Autodesk Inventor part; units mm, degrees
ref_plane "YZ Plane" through (0, 0, 0) normal (1, 0, 0) x (0, 1, 0)
ref_plane "XZ Plane" through (0, 0, 0) normal (0, 1, 0) x (-1, 0, 0)
ref_plane "XY Plane" through (0, 0, 0) normal (0, 0, 1) x (1, 0, 0)
sketch "Sketch1" plane through (0, 0, 0) normal (0, 0, 1) x (1, 0, 0)
  circle A0 centre (0, 0) radius 5
  arc A1 (-13, 15) -> (-15, 13) centre (-13, 13) ccw
  arc A2 (-15, -13) -> (-13, -15) centre (-13, -13) ccw
  arc A3 (13, -15) -> (15, -13) centre (13, -13) ccw
  arc A4 (15, 13) -> (13, 15) centre (13, 13) ccw
  arc A5 (-13, 14) -> (-14, 13) centre (-13, 13) ccw
  arc A6 (-14, -13) -> (-13, -14) centre (-13, -13) ccw
  arc A7 (13, -14) -> (14, -13) centre (13, -13) ccw
  arc A8 (14, 13) -> (13, 14) centre (13, 13) ccw
  line L0 (14, -14) -> (-14, 14) construction
  line L1 (-14, -14) -> (14, 14) construction
  line L2 (15, -15) -> (-15, 15) construction
  line L3 (-15, -15) -> (15, 15) construction
  line L4 (-13, 15) -> (-8, 15)
  line L5 (-8, 13) -> (-8, 8) construction
  line L6 (-9.4142, 8) -> (-13, 8)
  line L7 (-15, 8) -> (-15, 13)
  line L8 (-13, -15) -> (-8, -15)
  line L9 (-8, -13) -> (-8, -9.4142)
  line L10 (-9.4142, -8) -> (-13, -8)
  line L11 (-15, -8) -> (-15, -13)
  line L12 (13, -15) -> (8, -15)
  line L13 (8, -13) -> (8, -9.4142)
  line L14 (9.4142, -8) -> (13, -8)
  line L15 (15, -8) -> (15, -13)
  line L16 (13, 15) -> (8, 15)
  line L17 (8, 13) -> (8, 9.4142)
  line L18 (9.4142, 8) -> (13, 8)
  line L19 (15, 8) -> (15, 13)
  line L20 (-13, 9) -> (-10, 9)
  line L21 (-9, 10) -> (-9, 13)
  line L22 (-10, 14) -> (-13, 14)
  line L23 (-14, 13) -> (-14, 10)
  line L24 (13, 9) -> (10, 9)
  line L25 (9, 10) -> (9, 13)
  line L26 (10, 14) -> (13, 14)
  line L27 (14, 13) -> (14, 10)
  line L28 (13, -9) -> (10, -9)
  line L29 (9, -10) -> (9, -13)
  line L30 (10, -14) -> (13, -14)
  line L31 (14, -13) -> (14, -10)
  line L32 (-13, -9) -> (-10, -9)
  line L33 (-9, -10) -> (-9, -13)
  line L34 (-10, -14) -> (-13, -14)
  line L35 (-14, -13) -> (-14, -10)
  line L36 (-14, 13) -> (-14, 10)
  line L37 (-14, -10) -> (-14, -13)
  line L38 (-14, -13) -> (-14, -10)
  line L39 (-14, 10) -> (-14, 13)
  line L40 (13, -15) -> (5, -15)
  line L41 (-5, -15) -> (-13, -15)
  line L42 (13, -15) -> (5, -15) construction
  line L43 (0, -15) -> (-13, -15) construction
  line L44 (4, -13) -> (8, -13)
  line L45 (-8, -13) -> (-4, -13)
  line L46 (10, -9) -> (13, -9)
  line L47 (14, -10) -> (14, -13)
  line L48 (13, -14) -> (10, -14)
  line L49 (9, -13) -> (9, -10)
  line L50 (5, -14) -> (5, -15)
  line L51 (13, -14) -> (10, -14)
  line L52 (5, -14) -> (4, -14)
  line L53 (4, -14) -> (5, -14)
  line L54 (10, -14) -> (13, -14)
  line L55 (-4, -14) -> (-5, -14)
  line L56 (-10, -14) -> (-13, -14)
  line L57 (-13, -14) -> (-10, -14)
  line L58 (-5, -14) -> (-4, -14)
  line L59 (14, -13) -> (14, -10)
  line L60 (14, 10) -> (14, 13)
  line L61 (14, 13) -> (14, 10)
  line L62 (14, -10) -> (14, -13)
  line L63 (-5, -14) -> (-5, -15)
  line L64 (10, 14) -> (13, 14)
  line L65 (13, 14) -> (10, 14)
  line L66 (-10, 14) -> (-13, 14)
  line L67 (-13, 14) -> (-10, 14)
  line L68 (-5, 15) -> (-5, 14)
  line L69 (-13, 15) -> (-5, 15)
  line L70 (5, 15) -> (13, 15)
  line L71 (-15, 15) -> (-5, 15) construction
  line L72 (5, 15) -> (15, 15) construction
  line L73 (5, 15) -> (5, 14)
  line L74 (8, 13) -> (4, 13)
  line L75 (5, 14) -> (4, 14)
  line L76 (-5, 14) -> (-4, 14)
  line L77 (4, 14) -> (5, 14)
  line L78 (-4, 13) -> (-8, 13)
  line L79 (-4, 14) -> (-5, 14)
  line L80 (4, 13) -> (4, 14)
  line L81 (-4, 13) -> (-4, 14)
  line L82 (-4, -14) -> (-4, -13)
  line L83 (4, -14) -> (4, -13)
  line L84 (-8, 9.4142) -> (-4.1919, 5.6061)
  line L85 (8, 9.4142) -> (4.1919, 5.6061)
  line L86 (9.4142, 8) -> (5.6061, 4.1919)
  line L87 (5.6061, -4.1919) -> (9.4142, -8)
  line L88 (4.1919, -5.6061) -> (8, -9.4142)
  line L89 (-4.1919, -5.6061) -> (-8, -9.4142)
  line L90 (-5.6061, -4.1919) -> (-9.4142, -8)
  line L91 (-9.4142, 8) -> (-5.6061, 4.1919)
  arc A9 (4.1919, 5.6061) -> (-4.1919, 5.6061) centre (0, 0) ccw
  arc A10 (5.6061, -4.1919) -> (5.6061, 4.1919) centre (0, 0) ccw
  arc A11 (-5.6061, 4.1919) -> (-5.6061, -4.1919) centre (0, 0) ccw
  arc A12 (-4.1919, -5.6061) -> (4.1919, -5.6061) centre (0, 0) ccw
  line L92 (-8, 13) -> (-8, 9.4142)
  line L93 (-15, -13) -> (-15, -5) construction
  line L94 (-15, -13) -> (-15, -5)
  line L95 (-15, 5) -> (-15, 13)
  line L96 (15, -5) -> (15, -13) construction
  line L97 (15, 13) -> (15, 5)
  line L98 (15, -5) -> (15, -13)
  line L99 (-14, -4) -> (-14, -5)
  line L100 (14, -4) -> (14, -5)
  line L101 (14, 4) -> (14, 5)
  line L102 (-14, 4) -> (-14, 5)
  line L103 (-13, 8) -> (-13, 4)
  line L104 (13, 4) -> (13, 8)
  line L105 (13, -8) -> (13, -4)
  line L106 (-13, -4) -> (-13, -8)
  line L107 (-14, -5) -> (-15, -5)
  line L108 (15, -5) -> (14, -5)
  line L109 (15, 5) -> (14, 5)
  line L110 (-14, 5) -> (-15, 5)
  line L111 (13, 4) -> (14, 4)
  line L112 (-14, 4) -> (-13, 4)
  line L113 (-14, -4) -> (-13, -4)
  line L114 (13, -4) -> (14, -4)
  arc A13 (-13, -9) -> (-14, -10) centre (-13, -10) ccw
  arc A14 (-9, -10) -> (-10, -9) centre (-10, -10) ccw
  arc A15 (-10, -14) -> (-9, -13) centre (-10, -13) ccw
  arc A16 (10, -9) -> (9, -10) centre (10, -10) ccw
  arc A17 (9, -13) -> (10, -14) centre (10, -13) ccw
  arc A18 (14, -10) -> (13, -9) centre (13, -10) ccw
  arc A19 (10, 14) -> (9, 13) centre (10, 13) ccw
  arc A20 (9, 10) -> (10, 9) centre (10, 10) ccw
  arc A21 (13, 9) -> (14, 10) centre (13, 10) ccw
  arc A22 (-9, 13) -> (-10, 14) centre (-10, 13) ccw
  arc A23 (-10, 9) -> (-9, 10) centre (-10, 10) ccw
  arc A24 (-14, 10) -> (-13, 9) centre (-13, 10) ccw
  point P0 (15, -15)
  point P1 (-5.5858, -7)
  dimension "d0" = 30
  dimension "d1" = 30
  dimension "d2" = 10
  dimension "d4" = 2
  dimension "d11" = 28
  dimension "d12" = 7
  dimension "d13" = 7
  dimension "d15" = 1
  dimension "d16" = 1
  dimension "d17" = 1
  dimension "d18" = 1
  dimension "d19" = 5
  dimension "d23" = 30
  dimension "d27" = 1
  dimension "d30" = 3.5858
  dimension "d31" = 2
  dimension "d32" = 16
  dimension "d33" = 8
  dimension "d34" = 6
  dimension "d35" = 5.5858
extrude "Extrusion1" add sketch "Sketch1" along normal mid plane 97.1
sketch "Sketch3" plane through (-13, -15, 48.55) normal (0, -1, 0) x (1, 0, 0)
  line L0 (18, -97.1) -> (8, -97.1)
  line L1 (0, -97.1) -> (-1, -97.1)
  line L2 (-1, -97.1) -> (0, -97.1)
  line L3 (0, -97.1) -> (3, -97.1)
  line L4 (3, -97.1) -> (4, -97.1)
  line L5 (4, -97.1) -> (3, -97.1)
  line L6 (3, -97.1) -> (0, -97.1)
  line L7 (26, -97.1) -> (23, -97.1)
  line L8 (23, -97.1) -> (22, -97.1)
  line L9 (22, -97.1) -> (23, -97.1)
  line L10 (23, -97.1) -> (26, -97.1)
  line L11 (26, -97.1) -> (27, -97.1)
  line L12 (27, -97.1) -> (26, -97.1)
  line L13 (4, -97.1) -> (3, -97.1)
  line L14 (3, -97.1) -> (0, -97.1)
  line L15 (0, -97.1) -> (-1, -97.1)
  line L16 (-1, -97.1) -> (0, -97.1)
  line L17 (0, -97.1) -> (3, -97.1)
  line L18 (3, -97.1) -> (4, -97.1)
  line L19 (23, -97.1) -> (22, -97.1)
  line L20 (22, -97.1) -> (23, -97.1)
  line L21 (23, -97.1) -> (26, -97.1)
  line L22 (26, -97.1) -> (27, -97.1)
  line L23 (27, -97.1) -> (26, -97.1)
  line L24 (26, -97.1) -> (23, -97.1)
  line L25 (5, -97.1) -> (8.8081, -97.1)
  line L26 (8.8081, -97.1) -> (17.1919, -97.1)
  line L27 (17.1919, -97.1) -> (21, -97.1)
  line L28 (21, -97.1) -> (17, -97.1)
  line L29 (17, -97.1) -> (18, -97.1)
  line L30 (18, -97.1) -> (26, -97.1)
  line L31 (26, -97.1) -> (28, -97.1)
  line L32 (28, -97.1) -> (27, -97.1)
  line L33 (27, -97.1) -> (26, -97.1)
  line L34 (26, -97.1) -> (22.4142, -97.1)
  line L35 (22.4142, -97.1) -> (18.6061, -97.1)
  line L36 (18.6061, -97.1) -> (18.6061, -97.1)
  line L37 (18.6061, -97.1) -> (22.4142, -97.1)
  line L38 (22.4142, -97.1) -> (26, -97.1)
  line L39 (26, -97.1) -> (27, -97.1)
  line L40 (27, -97.1) -> (28, -97.1)
  line L41 (28, -97.1) -> (26, -97.1)
  line L42 (26, -97.1) -> (18, -97.1)
  line L43 (18, -97.1) -> (17, -97.1)
  line L44 (17, -97.1) -> (21, -97.1)
  line L45 (21, -97.1) -> (17.1919, -97.1)
  line L46 (17.1919, -97.1) -> (8.8081, -97.1)
  line L47 (8.8081, -97.1) -> (5, -97.1)
  line L48 (5, -97.1) -> (9, -97.1)
  line L49 (9, -97.1) -> (8, -97.1)
  line L50 (8, -97.1) -> (0, -97.1)
  line L51 (0, -97.1) -> (-2, -97.1)
  line L52 (-2, -97.1) -> (-1, -97.1)
  line L53 (-1, -97.1) -> (0, -97.1)
  line L54 (0, -97.1) -> (3.5858, -97.1)
  line L55 (3.5858, -97.1) -> (7.3939, -97.1)
  line L56 (7.3939, -97.1) -> (7.3939, -97.1)
  line L57 (7.3939, -97.1) -> (3.5858, -97.1)
  line L58 (3.5858, -97.1) -> (0, -97.1)
  line L59 (0, -97.1) -> (-1, -97.1)
  line L60 (-1, -97.1) -> (-2, -97.1)
  line L61 (-2, -97.1) -> (0, -97.1)
  line L62 (0, -97.1) -> (8, -97.1)
  line L63 (8, -97.1) -> (9, -97.1)
  line L64 (9, -97.1) -> (5, -97.1)
  line L65 (39.4927, -105.2765) -> (-27.442, -57.6557)
  line L66 (-27.442, -57.6557) -> (-27.442, -105.2765)
  line L67 (27, -97.1) -> (27, 0)
  line L68 (-27.442, -105.2765) -> (39.4927, -105.2765)
  point P0 (13, -48.55)
  dimension "d36" = 35.43
extrude "Extrusion2" cut sketch "Sketch3" against normal blind 30
properties part number "pole_supoort_1" material "Aluminum 6061"
Check sheet for the modelled part. Datum: model origin and axes. Units: mm. A direction names the side the tool comes from. Coordinates: 2 decimals unless noted, no trailing zeros. Write each loop counter-clockwise with the first axis right and the second up, starting at its lowest first coordinate (ties: lowest second). Pieces come first, ordered by that corner, then holes. Notation, with made-up numbers: M 20,-6 L 28,-6 A14 ccw 28,17 Z; hole C -32.75,22 d10. An arc over 180 degrees is marked long. Write item = value, one per line. Start each with the question number.
1. Mould release check, pull along X, two halves, no side actions. Record for faces 3 (the flat face through (9, 15, 0)), 4 (the cylindrical face through (4.77, -1.5, 2.93)), 5 (the cylindrical face through (14.43, -14.4, -0.68)), 6 (the cylindrical face through (-14.4, -14.43, 9.42)): pulls with the +X half, pulls with the -X half, needs draft (parallel to the pull), parting line crosses it, or undercut.
2. Tool access check on faces 1 (the flat face through (8, -11, 2)), 2 (the flat face through (-9, -15, 7)). Record the directions out of +Z, -Z, +X, -X, +Y, -Y that give a thin tool (end or side, any length) a straight path to the whole face; none if there is none.
3. Sectioned sample at C-C (x = 2). Record the cut outline in (y, z), then the cut area to 3 significant figures.
4. Sectioned sample at B-B (x = 12). Record the cut outline in (y, z).
5. Thickness scan on probe 1 along X at (y, z) = (0, -17); probe 2 along X at (y, z) = (-5.75, -29.5). Record the ranges inside material, lowest first.
6. Sectioned sample at A-A (y = 3). Record the cut outline in (x, z), then the cut area to 3 significant figures.
7. Sectioned sample at D-D (z = 41). State how many separate pieces and enclosed holes the cut face has, then the cut area to 3 significant figures.
8. Go/stop test with flat-tipped pins: pin 1 (0.5 mm diameter, centred on y = -13.5, z = -12.5, fed in from -X); pin 2 (0.8 mm diameter, centred on x = -14.5, z = 8, fed in from +Y); pin 3 (1.1 mm diameter, centred on x = -14.5, z = 6.5, fed in from -Y). Record where each tip stops, or that it passes through.
The answers:
q1.face_3 = needs draft
q1.face_4 = undercut
q1.face_5 = pulls with the +X half
q1.face_6 = pulls with the -X half
q2.face_1 = +Z, -Z
q2.face_2 = +Z, -Z, +X, -X, -Y
q3.outline = M -6.71,-39.3 L -4.58,-39.3 L -4.58,48.55 L -6.71,48.55 Z; M 4.58,-39.3 L 6.71,-39.3 L 6.71,48.55 L 4.58,48.55 Z
q3.area = 373 mm²
q4.outline = M -15,-46.42 L -14,-46.42 L -14,48.55 L -15,48.55 Z; M -9,-46.42 L -8,-46.42 L -8,48.55 L -9,48.55 Z; M 8,-46.42 L 9,-46.42 L 9,48.55 L 8,48.55 Z; M 14,-46.42 L 15,-46.42 L 15,48.55 L 14,48.55 Z
q5.probe_1 = -7 to -5, 5 to 7
q5.probe_2 = -7.16 to -4.34, -3.99 to 3.99, 4.34 to 7.16, 13 to 15
q6.outline = M -6.32,-33.38 L -4,-35.03 L -4,48.55 L -6.32,48.55 Z; M 4,-40.72 L 6.32,-42.38 L 6.32,48.55 L 4,48.55 Z
q6.area = 402 mm²
q7.separate_pieces = 1
q7.enclosed_holes = 5
q7.area = 266 mm²
q8.pin_1 = -14.98
q8.pin_2 = 14.67
q8.pin_3 = -14.76
